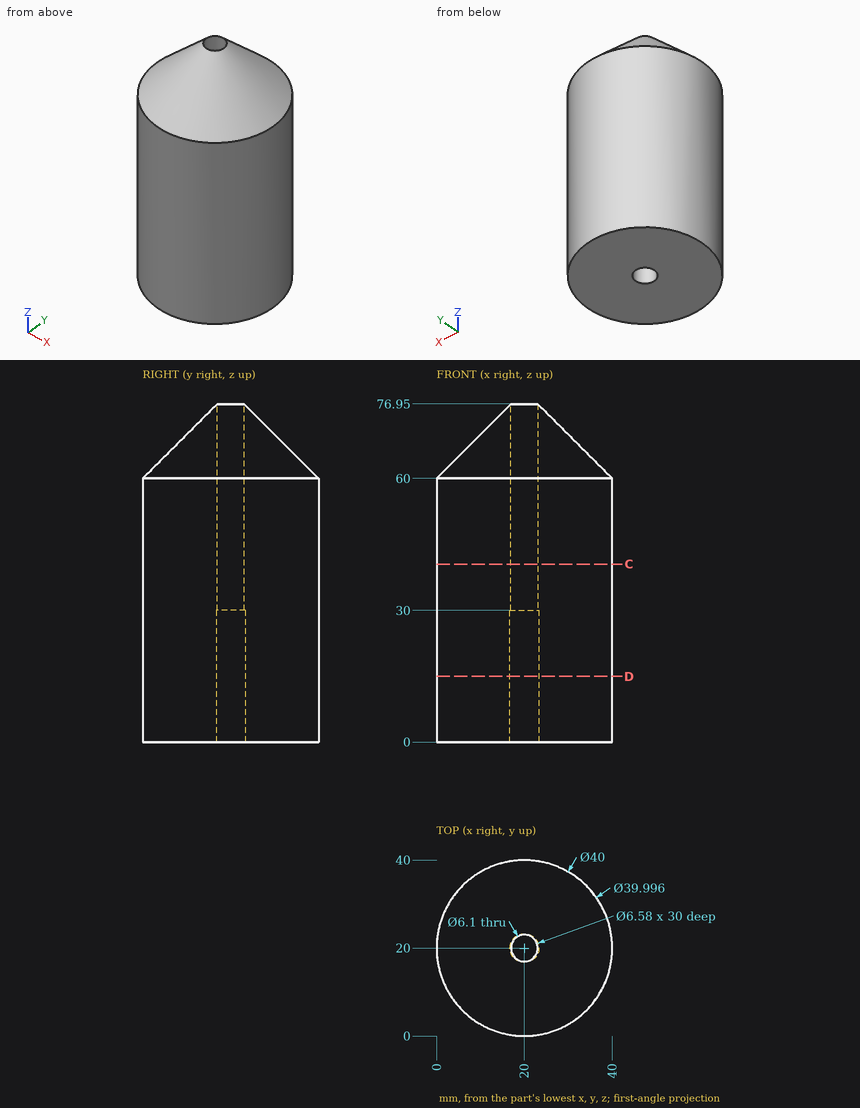
Geometry check sheet. Reference: drawing and pictorial views, mm from the part's lowest x, y, z. Give positions to 0.01 mm unless a question says otherwise; leave off trailing zeros. Loops run counter-clockwise (first coordinate to the right, second up) from the corner with the lowest first, then second, coordinate; pieces in that order, holes last. Notation, with made-up numbers: M -18,82 L 8,82 A27 ccw 8,102 Z; hole C 19,48.5 d10. An arc over 180 degrees is marked long. Use a Markdown table: item, result. Add a question column.
Q1. Scan lines: line 1 along Y through (x, z) = (20, 10.5); line 2 along Y through (x, z) = (21.5, 49.5) (1 decimal); line 3 along X through (y, z) = (22, 72.5). Record each from-to range of solid material in increasing order. Write a range as [from, to].
Q2. Go/stop test with flat-tipped pins: pin 1 (8 mm diameter, centred on x = 36, z = 65.5, fed in from -Y) (1 decimal); pin 2 (8 mm diameter, centred on x = 33, z = 37, fed in from +Y); pin 3 (10 mm diameter, centred on x = 9, z = 26, fed in from -Y); pin 4 (3.5 mm diameter, centred on x = 20, y = 20, fed in from -Z). Record where each tip stops, or that it passes through.
Q3. Sectioned sample at D-D, the plane z = 15. Record the cut outline in (x, y), then the cut area to 3 significant figures.
Q4. Sectioned sample at C-C, the plane z = 40.5. Record the cut outline in (x, y).
Verdict:
| question | item | result |
|---|---|---|
| 1 | line 1 | [0, 16.71], [23.29, 40] |
| 1 | line 2 | [0.1, 17.3], [22.7, 39.9] |
| 1 | line 3 | [12.77, 17.7], [22.3, 27.23] |
| 2 | pin 1 | y = 8.7 |
| 2 | pin 2 | y = 37.86 |
| 2 | pin 3 | y = 0.92 |
| 2 | pin 4 | through |
| 3 | outline | C 20,20 d40; hole C 20,20 d6.58 |
| 3 | area | 1,220 mm^2 |
| 4 | outline | C 20,20 d40; hole C 20,20 d6.1 |
